Design review of the part built by this model. Coordinates are the model's own, in mm. Face numbers are marked on the shaded views. A direction names the side the tool comes from. Coordinates: 2 decimals unless noted, no trailing zeros. Loops run counter-clockwise (first coordinate to the right, second up) from the corner with the lowest first, then second, coordinate; pieces in that order, holes last. Notation, with made-up numbers: (66.5, -24) -> (123.5, -24) arc R26 ccw to (123.5, 11) -> close; hole circle Ø1 at (11.5, 83.5). An arc over 180 degrees is marked (long way). Answer as a JSON object with one key per item and string values.
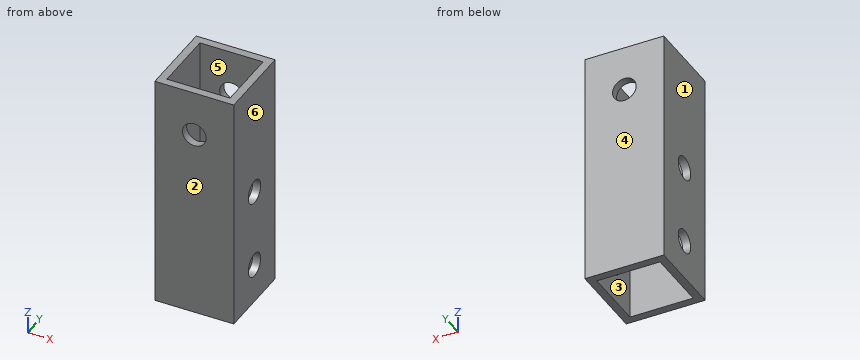
```python
from build123d import *

# Parameters (mm, degrees)
SKETCH_1_W          = 10
SKETCH_1_H          = 10
SKETCH_1_W_2        = 8
SKETCH_1_H_2        = 8
EXTRUDE_1_DEPTH     = 30
SKETCH_2_R          = 1.5
CUT_EXTRUDE_1_DEPTH = 11
SKETCH_3_R          = 1.5
CUT_EXTRUDE_2_DEPTH = 11


with BuildPart() as part:
    # 草图1 → 拉伸-薄壁1 (new body)
    with BuildSketch(Plane.XY):
        Rectangle(SKETCH_1_W, SKETCH_1_H)
        Rectangle(SKETCH_1_W_2, SKETCH_1_H_2, mode=Mode.SUBTRACT)
    extrude(amount=EXTRUDE_1_DEPTH)

    # 草图2 → 切除-拉伸1 (cut, through all)
    with BuildSketch(Plane(origin=(5, 0, 0), x_dir=(0, 0, -1), z_dir=(1, 0, 0))):
        with Locations((-5, 0)):
            Circle(SKETCH_2_R)
        with Locations((-15, 0)):
            Circle(SKETCH_2_R)
    extrude(amount=-CUT_EXTRUDE_1_DEPTH, mode=Mode.SUBTRACT)

    # 草图3 → 切除-拉伸2 (cut, through all)
    with BuildSketch(Plane(origin=(0, 5, 0), x_dir=(1, 0, 0), z_dir=(0, 1, 0))):
        with Locations((0, -24.3)):
            Circle(SKETCH_3_R)
    extrude(amount=-CUT_EXTRUDE_2_DEPTH, mode=Mode.SUBTRACT)


solid = part.part
```
1) Add section A-A, the plane x = 2.75. Give the boundary of the cut face in (y, z).
Completed:
{"outline": "(-5, 0) -> (-4, 0) -> (-4, 30) -> (-5, 30) -> close; (4, 0) -> (5, 0) -> (5, 30) -> (4, 30) -> close"}
2) Add section C-C, the plane z = 25.5. Give the boundary of the cut face in (x, y).
Completed:
{"outline": "(-5, -5) -> (-0.9, -5) -> (-0.9, -4) -> (-4, -4) -> (-4, 4) -> (-0.9, 4) -> (-0.9, 5) -> (-5, 5) -> close; (0.9, -5) -> (5, -5) -> (5, 5) -> (0.9, 5) -> (0.9, 4) -> (4, 4) -> (4, -4) -> (0.9, -4) -> close"}
3) Wall thickness on probe 1 along Y at (x, z) = (4.55, 15); probe 2 along X at (y, z) = (2.25, 26.25): over which ranges is each line inside the solid? List them lowest first.
Completed:
{"probe 1": "-5 to -1.5, 1.5 to 5", "probe 2": "-5 to -4, 4 to 5"}
4) For the marked faces 5 and 6, list the 3-axis set-ups (+Z, -Z, +X, -X, +Y, -Y) from which the entire face can be reached by the end or side of a thin tool; tool diameter is ignored.
Completed:
{"face 5": "+Z, -Z", "face 6": "+Z, -Z, +X, +Y, -Y"}
5) The part is to be moulded in two halves that separate along Y. For the marked faces 1, 2, 3 and 4, say which applies: pulls with the +Y half, pulls with the -Y half, needs draft (parallel to the pull), parting line crosses it, or undercut.
Completed:
{"face 1": "needs draft", "face 2": "pulls with the -Y half", "face 3": "undercut", "face 4": "pulls with the +Y half"}
6) Add section D-D, the plane x = 0. Give the boundary of the cut face in (y, z).
Completed:
{"outline": "(-5, 0) -> (-4, 0) -> (-4, 22.8) -> (-5, 22.8) -> close; (-5, 25.8) -> (-4, 25.8) -> (-4, 30) -> (-5, 30) -> close; (4, 0) -> (5, 0) -> (5, 22.8) -> (4, 22.8) -> close; (4, 25.8) -> (5, 25.8) -> (5, 30) -> (4, 30) -> close"}
7) Clearance check with a flat-ended pin moving along its axis: pin 1 Ø2 at (x, y) = (-2, -1) entering from -Z. State where the tip first meets the part, or that it passes through.
Completed:
{"pin 1": "through"}
